Check sheet for the modelled part. Datum: model origin and axes. Units: mm. A direction names the side the tool comes from. Give positions to 0.01 mm unless a question says otherwise; leave off trailing zeros. Order: outer loops, then holes, each group sorted by start corner. A loop starts at its lowest first (then second) coordinate and runs counter-clockwise, first axis right, second up. Notation, with made-up numbers: (79, 33.5) -> (130, 33.5) arc R14 ccw to (130, 38.5) -> close; hole circle Ø8 at (17, 84). An arc over 180 degrees is marked (long way). Answer in a Markdown table with one row per item. Add a question column.
(1) Cross-section at B-B (z = 5.75). Record the cut outline in (x, y).
(2) Cross-section at C-C (x = -9.5). Record the cut outline in (y, z), then the cut area to 3 significant figures.
(3) Set-up check for faces 4 (the face through (8.688, 1.525, 16.09)), 5 (the face through (-9, 0, 14)), 6 (the face through (9, -1, 15)): record each of +Z, -Z, +X, -X, +Y, -Y from which the full face is reachable in a straight line by a thin tool's end or side.
(4) Go/stop test with flat-tipped pins: pin 1 (1.4 mm diameter, centred on x = 12, y = 0.5, fed in from -Z); pin 2 (2 mm diameter, centred on y = 0.5, z = 15, fed in from -X); pin 3 (1.8 mm diameter, centred on y = 0, z = 15, fed in from +X); pin 4 (1 mm diameter, centred on y = -1, z = 26.5, fed in from -X). Record where each tip stops, or that it passes through.
(5) Release check for a two-part mould opening along Z. For faces 1 (the face through (2.279, 0, 6)), 2 (the face through (8.69, 1.55, 14.17)), 3 (the face through (9, 0, 18)) record: released by +Z, released by -Z, zero draft, split by the parting line, or undercut.
(6) Cross-section at D-D (x = 9). Record the cut outline in (y, z), then the cut area to 3 significant figures.
(7) Thickness scan on L1, parallel to Z at x = -9, y = 0; L2, parallel to X at y = 0, z = 19.5; L3, parallel to X at y = 0, z = 12.5. Record the ranges inside material, lowest first. Write a range as [from, to].
(8) Cross-section at A-A (y = -0.4). Record the cut outline in (x, z), then the cut area to 3 significant figures.
```python
from build123d import *

# Parameters (mm, degrees)
F1_DEPTH = 30
F3_DEPTH = 13
F4_W     = 4.553619
F4_H     = 6
F4_R     = 1
F5_DEPTH = 13


with BuildPart() as f1:
    # F0 (on Top) → F1 (new body)
    with BuildSketch(Plane.XY):
        with BuildLine():
            ThreePointArc((0.8, 1.024695), (1.168332, 0.570088), (1.3, 0))
            ThreePointArc((1.3, 0), (-0.570088, -1.168332), (-0.8, 1.024695))
            Line((-0.8, 1.024695), (-1, 2.015564))
            ThreePointArc((-1, 2.015564), (-1.185854, -1.912132), (2.25, 0))
            ThreePointArc((2.25, 0), (1.912132, 1.185854), (1, 2.015564))
            Line((1, 2.015564), (0.8, 1.024695))
        make_face()
        with BuildLine():
            Line((1.047319, 2.25), (1, 2.015564))
            ThreePointArc((1, 2.015564), (1.912132, 1.185854), (2.25, 0))
            ThreePointArc((2.25, 0), (-1.185854, -1.912132), (-1, 2.015564))
            Line((-1, 2.015564), (-1.047319, 2.25))
            Line((-1.047319, 2.25), (-2.274133, 2.25))
            Line((-2.274133, 2.25), (-2.274133, -2.303619))
            Line((-2.274133, -2.303619), (2.279486, -2.303619))
            Line((2.279486, -2.303619), (2.279486, 2.25))
            Line((2.279486, 2.25), (1.047319, 2.25))
        make_face()
    extrude(amount=F1_DEPTH)

    # F2 (on face) → F3 (join)
    with BuildSketch(Plane.YZ.offset(2.279486)):
        with BuildLine():
            ThreePointArc((0.824123, 14.433589), (-0.999993, 14.996283), (0.819889, 15.572522))
            Line((0.819889, 15.572522), (2.25, 16.621344))
            Line((2.25, 16.621344), (2.25, 18))
            Line((2.25, 18), (-2.303619, 18))
            Line((-2.303619, 18), (-2.303619, 12))
            Line((-2.303619, 12), (2.25, 12))
            Line((2.25, 12), (2.25, 13.912768))
            Line((2.25, 13.912768), (0.824123, 14.433589))
        make_face()
    extrude(amount=F3_DEPTH)

    # F4 (on face) → F5 (join)
    with BuildSketch(Plane(origin=(-2.274133, 0, 0), x_dir=(0, -1, 0), z_dir=(-1, 0, 0))):
        with Locations((0.026809, 15)):
            Rectangle(F4_W, F4_H)
        with Locations((0, 15)):
            Circle(F4_R, mode=Mode.SUBTRACT)
    extrude(amount=F5_DEPTH)


solid = f1.part
```
Answer below:
| question | item | result |
|---|---|---|
| 1 | outline | (-2.27, -2.3) -> (2.28, -2.3) -> (2.28, 2.25) -> (1.05, 2.25) -> (1, 2.02) -> (0.8, 1.02) arc R1.3 cw (long way) to (-0.8, 1.02) -> (-1, 2.02) -> (-1.05, 2.25) -> (-2.27, 2.25) -> close |
| 2 | outline | (-2.3, 12) -> (2.25, 12) -> (2.25, 18) -> (-2.3, 18) -> close; hole circle Ø2 at (0, 15) |
| 2 | area | 24.2 mm² |
| 3 | face 4 | +X, +Y |
| 3 | face 5 | -X |
| 3 | face 6 | +X |
| 4 | pin 1 | stops at z = 12 |
| 4 | pin 2 | stops at x = -15.27 |
| 4 | pin 3 | stops at x = 2.28 |
| 4 | pin 4 | stops at x = -2.27 |
| 5 | face 1 | zero draft |
| 5 | face 2 | undercut |
| 5 | face 3 | released by +Z |
| 6 | outline | (-2.3, 12) -> (2.25, 12) -> (2.25, 13.91) -> (0.82, 14.43) arc R1 cw (long way) to (0.82, 15.57) -> (2.25, 16.62) -> (2.25, 18) -> (-2.3, 18) -> close |
| 6 | area | 21.6 mm² |
| 7 | L1 | z = [12, 14], [16, 18] |
| 7 | L2 | x = [-2.27, -1.3], [1.3, 2.28] |
| 7 | L3 | x = [-15.27, -1.3], [1.3, 15.28] |
| 8 | outline | (-15.27, 12) -> (-2.27, 12) -> (-2.27, 0) -> (-1.24, 0) -> (-1.24, 30) -> (-2.27, 30) -> (-2.27, 18) -> (-15.27, 18) -> (-15.27, 15.92) -> (-2.27, 15.92) -> (-2.27, 14.08) -> (-15.27, 14.08) -> close; (1.24, 0) -> (2.28, 0) -> (2.28, 12) -> (15.28, 12) -> (15.28, 14.08) -> (2.28, 14.08) -> (2.28, 15.92) -> (15.28, 15.92) -> (15.28, 18) -> (2.28, 18) -> (2.28, 30) -> (1.24, 30) -> close |
| 8 | area | 171 mm² |
